Source: CAD feature listing. Evaluate the final solid. Frame: model axes, mm. Round coordinates to 2 decimals unless told otherwise and drop trailing zeros. Write each loop counter-clockwise with the first axis right and the second up, starting at its lowest first coordinate (ties: lowest second). Pieces come first, ordered by that corner, then holes. Notation, with made-up numbers: (42, -0.5) -> (91, -0.5) arc R21 cw to (91, 6.5) -> close; hole circle Ø4 at (39, 12). An arc over 180 degrees is marked (long way). Put each result on its own line as item: value.
```python
from build123d import *

# Parameters (mm, degrees)
SKETCH2_W            = 558.8
SKETCH2_H            = 38.1
SKETCH2_R            = 6.35
MOWER_BLADE_DEPTH    = 3.175
CUTTING_EDGE_1_DEPTH = 101.6
CUTTING_EDGE_2_DEPTH = 101.6


with BuildPart() as part:
    # Sketch2 → Mower Blade (new body)
    with BuildSketch(Plane(origin=(0, 0, 0), x_dir=(1, 0, 0), z_dir=(0, 1, 0))):
        Rectangle(SKETCH2_W, SKETCH2_H)
        Circle(SKETCH2_R, mode=Mode.SUBTRACT)
    extrude(amount=MOWER_BLADE_DEPTH)

    # Sketch3 → Cutting Edge #1 (cut)
    with BuildSketch(Plane(origin=(279.4, 0, 0), x_dir=(0, 0, -1), z_dir=(1, 0, 0))):
        Polygon((19.05, 0), (11.43, 3.175), (19.05, 3.175), align=None)
    extrude(amount=-CUTTING_EDGE_1_DEPTH, mode=Mode.SUBTRACT)

    # Sketch4 → Cutting Edge #2 (cut)
    with BuildSketch(Plane.ZY.offset(279.4)):
        Polygon((19.05, 0), (11.43, 3.175), (19.05, 3.175), align=None)
    extrude(amount=-CUTTING_EDGE_2_DEPTH, mode=Mode.SUBTRACT)


solid = part.part
```
Q1. Cut plane A-A on x = 0. Output: boundary loops of the cut face in (y, z) (3 decimals), and give its area (3 significant figures).
Ans:
outline: (0, -19.05) -> (3.175, -19.05) -> (3.175, -6.35) -> (0, -6.35) -> close; (0, 6.35) -> (3.175, 6.35) -> (3.175, 19.05) -> (0, 19.05) -> close
area: 80.6 mm^2
Q2. Cut plane C-C on y = 1. Output: boundary loops of the cut face in (x, z), and give its area (3 significant figures).
Ans:
outline: (-279.4, -19.05) -> (177.8, -19.05) -> (177.8, -16.65) -> (279.4, -16.65) -> (279.4, 19.05) -> (-177.8, 19.05) -> (-177.8, 16.65) -> (-279.4, 16.65) -> close; hole circle Ø12.7 at (0, 0)
area: 20,700 mm^2
Q3. Cut plane B-B on z = 0. Output: boundary loops of the cut face in (x, y) (3 decimals).
Ans:
outline: (-279.4, 0) -> (-6.35, 0) -> (-6.35, 3.175) -> (-279.4, 3.175) -> close; (6.35, 0) -> (279.4, 0) -> (279.4, 3.175) -> (6.35, 3.175) -> close
Q4. Draft query along X for faces 1 (the flat face through (-4, 3.175, -9)), 2 (the cylindrical face through (-1.38, 1.57, 6.2)). Return one class per face: +X half, -X half, draft (parallel to the pull), parting line (faces both ways), or undercut.
Ans:
face 1: draft
face 2: undercut
Q5. Pin query (flat end, axial travel): pin 1 (4 mm diameter, centred on x = -92.5, z = 0.5, fed in from -Y). Return the tip coordinate at first contact, or that it passes through.
Ans:
pin 1: stops at y = 0
Q6. Material intervals for line 1 (Z direction, x = 0, y = 2.5); line 2 (X direction, y = 2.2, z = 0); line 3 (Z direction, x = -219, y = 1.3), sorted ascending. Write a range as [from, to].
Ans:
line 1: z = [-19.05, -6.35], [6.35, 19.05]
line 2: x = [-279.4, -6.35], [6.35, 279.4]
line 3: z = [-19.05, 15.93]
